Part model, mm, in its own coordinate system. A direction names the side the tool comes from. Give positions to 0.01 mm unless a question says otherwise; leave off trailing zeros. Order: outer loops, then holes, each group sorted by start corner. A loop starts at its lowest first (then second) coordinate and runs counter-clockwise, first axis right, second up. Notation, with made-up numbers: (67.5, 15.25) - (93.5, 15.25) arc R9 cw to (93.5, 22.25) - close; hole circle Ø10 at (65, -10). An arc over 180 degrees is marked (long way). One line per item, written item: value.
Autodesk Inventor part; units mm, degrees
ref_plane "YZ Plane" through (0, 0, 0) normal (1, 0, 0) x (0, 1, 0)
ref_plane "XZ Plane" through (0, 0, 0) normal (0, 1, 0) x (-1, 0, 0)
ref_plane "XY Plane" through (0, 0, 0) normal (0, 0, 1) x (1, 0, 0)
sketch "Skizze1" plane through (0, 0, 0) normal (1, 0, 0) x (0, 1, 0)
  line L0 (0, 0) -> (28, 0)
  line L1 (28, 0) -> (28, -50)
  line L2 (28, -50) -> (0, -50)
  line L3 (0, -50) -> (0, 0)
  dimension "d0" = 28
  dimension "d1" = 50
extrude "Extrusion1" add sketch "Skizze1" along normal blind 17
shell "Wandung1" thickness 2 removed faces 1 at (17, 9.3333, -16.6667)
sketch "Skizze2" plane through (2, 2, -2) normal (1, 0, 0) x (0, 0, -1)
  circle A0 centre (35.75, 10.2) radius 8.2
  circle A1 centre (10.15, 10.2) radius 8.2
  line L0 (46, 0) -> (0, 0)
  line L1 (0, 0) -> (0, 24)
  point P0 (-2, -2)
  dimension "d5" = 16.4
  dimension "d9" = 25.6
  dimension "d10" = 10.15
  dimension "d11" = 10.2
extrude "Extrusion2" cut sketch "Skizze2" against normal blind 14
sketch "Skizze3" plane through (2, 2, -2) normal (1, 0, 0) x (0, 0, -1)
  line L0 (0, 24) -> (0, 0)
  line L1 (0, 0) -> (3, 0)
  line L2 (3, 0) -> (3, 3)
  line L3 (3, 3) -> (0, 3)
  line L4 (0, 3) -> (0, 0)
  line L5 (0, 0) -> (46, 0)
  line L6 (46, 0) -> (43, 0)
  line L7 (43, 0) -> (43, 3)
  line L8 (43, 3) -> (46, 3)
  line L9 (46, 3) -> (46, 0)
  line L10 (46, 0) -> (46, 24)
  line L11 (46, 20) -> (43, 20)
  line L12 (43, 20) -> (43, 17)
  line L13 (43, 17) -> (46, 17)
  line L14 (46, 17) -> (46, 20)
  line L15 (0, 20) -> (3, 20)
  line L16 (3, 20) -> (3, 17)
  line L17 (3, 17) -> (0, 17)
  line L18 (0, 17) -> (0, 20)
  point P0 (-2, -2)
  point P1 (43, 0)
  point P2 (0, 20)
  point P3 (0, 17)
  dimension "d14" = 3
  dimension "d15" = 3
  dimension "d16" = 3
  dimension "d17" = 3
  dimension "d18" = 3
  dimension "d19" = 20
extrude "Extrusion3" add sketch "Skizze3" along normal blind 4
fillet "Rundung1" radius 0.3 23 edges at (4, 19, -5) (4, 22, -5) (4, 19, -2) (4, 22, -2) (4, 5, -2) (4, 5, -5) (4, 2, -5) (4, 22, -45) (2, 3.5, -45) (2, 5, -46.5) (4, 5, -45) (2, 22, -3.5) (2, 20.5, -5) (2, 5, -3.5) (2, 3.5, -5) (4, 19, -45) (4, 22, -48) (4, 5, -48) (4, 2, -45) (2, 22, -46.5) (2, 20.5, -45) (2, 19, -46.5) (2, 19, -3.5)
sketch "Skizze4" plane through (2, 26, -48) normal (0, -1, 0) x (1, 0, 0)
  line L0 (12, 30) -> (5, 30)
  line L1 (5, 30) -> (5, 16.5)
  line L2 (5, 16.5) -> (12, 16.5)
  line L3 (12, 16.5) -> (12, 30)
  line L4 (4, 43.3) -> (4, 45.7)
  line L5 (0, 46) -> (15, 46)
  point P0 (-2, 48)
  dimension "d23" = 1
  dimension "d24" = 7
  dimension "d25" = 13.5
  dimension "d26" = 16
extrude "Extrusion4" cut sketch "Skizze4" against normal blind 17
properties part number "gehaeuse_hc-sr04"
1) Drill centre lines: line 1 along Y through (x, z) = (4, -45.5); line 2 along Y through (x, z) = (1.6, -12.15); line 3 along Z through (x, y) = (11, 4). Where is each one in solid material? Low to high. Write a range as from..to.
Outcome:
line 1: y = 0..5, 19..22, 26..28
line 2: y = 0..4, 20.4..28
line 3: z = -50..-48, -2..0
2) Cut at D-D, the plane z = -37.75. Give the cut face in (x, y), then the cut area to 3 significant figures.
Outcome:
outline: (0, 0) - (17, 0) - (17, 2) - (2, 2) - (2, 4) - (0, 4) - close; (0, 20.4) - (2, 20.4) - (2, 26) - (17, 26) - (17, 28) - (0, 28) - close
area: 83.2 mm^2
3) Mould opens along Z. For faces 1 (the flat face through (9, 14, -48)), 2 (the flat face through (8, 0, -25)), 3 (the flat face through (8, 14, 0)) say: released by +Z, released by -Z, zero draft, split by the parting line, or undercut.
Outcome:
face 1: undercut
face 2: zero draft
face 3: released by +Z
4) Cut at C-C, the plane x = 14.75. Give the cut face in (y, z).
Outcome:
outline: (0, -50) - (28, -50) - (28, 0) - (0, 0) - close; hole (2, -48) - (26, -48) - (26, -2) - (2, -2) - close
5) Which spindle directions (+Z, -Z, +X, -X, +Y, -Y) get a long thin tool onto all of the face, cutting with end or side? Do faces 4 (the flat face through (6, 4, -46)), 5 (the flat face through (14, 27, -25)), 6 (the cylindrical face through (1.014, 12.561, -29.558)). Say none if no direction does.
Outcome:
face 4: +X
face 5: +Y
face 6: +X, -X
6) Pin check, flat tips, straight feed: pin 1 (2 mm diameter, centred on x = 10.5, z = -20.5, fed in from +Y); pin 2 (0.7 mm diameter, centred on x = 4, y = 20.5, fed in from +Z); pin 3 (4 mm diameter, centred on y = 6, z = -10, fed in from +X); pin 4 (1.6 mm diameter, centred on y = 3, z = -46, fed in from +X). Stop position of each tip, or through.
Outcome:
pin 1: stops at y = 2
pin 2: stops at z = 0
pin 3: stops at x = 2
pin 4: stops at x = 6
7) Cut at B-B, the plane z = -16. Give the cut face in (x, y), then the cut area to 3 significant figures.
Outcome:
outline: (0, 0) - (17, 0) - (17, 2) - (2, 2) - (2, 4.96) - (0, 4.96) - close; (0, 19.44) - (2, 19.44) - (2, 26) - (17, 26) - (17, 28) - (0, 28) - close
area: 87.0 mm^2
8) Cut at A-A, the plane y = 12.2. Give the cut face in (x, z).
Outcome:
outline: (0, -50) - (17, -50) - (17, -48) - (2, -48) - (2, -45.95) - (0, -45.95) - close; (0, -29.55) - (2, -29.55) - (2, -20.35) - (0, -20.35) - close; (0, -3.95) - (2, -3.95) - (2, -2) - (17, -2) - (17, 0) - (0, 0) - close
